```python
from build123d import *

# Parameters (mm, degrees)
F0_R     = 1.524
F1_DEPTH = 3.175
F2_R     = 5.08


# Not quite as in the source:
# - a feature names something its author has since deleted; it is built from what else it names


with BuildPart() as f1:
    # F0 (on Top) → F1 (new body)
    with BuildSketch(Plane.XY):
        Polygon((-6.35, -25.4), (6.35, -25.4), (6.35, 25.4), (6.35, 76.2), (-6.35, 76.2), (-6.35, 25.4), align=None)
        with Locations((0, -19.05)):
            Circle(F0_R, mode=Mode.SUBTRACT)
        with Locations((0, 19.05)):
            Circle(F0_R, mode=Mode.SUBTRACT)
    extrude(amount=F1_DEPTH)

    # F2
    f2_edges = [f1.edges().sort_by_distance(p)[0] for p in [
        (-6.35, 76.2, 1.5875),
        (6.35, 76.2, 1.5875),
        (-6.35, -25.4, 1.5875),
        (6.35, -25.4, 1.5875),
    ]]
    fillet(f2_edges, radius=F2_R)


solid = f1.part
```
Input: part model. Units: mm. Frame: model coordinates. Give positions to 0.01 mm unless a question says otherwise; leave off trailing zeros. Order: outer loops, then holes, each group sorted by start corner. A loop starts at its lowest first (then second) coordinate and runs counter-clockwise, first axis right, second up. Notation, with made-up numbers: (60, 46) - (80, 46) arc R25 ccw to (80, 61) - close; hole circle Ø6 at (76, 22.25). An arc over 180 degrees is marked (long way). Use a Markdown table: item, result.
(1) Section query A-A (y = -19.05). Output: boundary loops of the cut face in (x, z) (3 decimals), then the cut area to 3 significant figures.
Computed values:
| item | result |
|---|---|
| outline | (-6.35, 0) - (-1.524, 0) - (-1.524, 3.175) - (-6.35, 3.175) - close; (1.524, 0) - (6.35, 0) - (6.35, 3.175) - (1.524, 3.175) - close |
| area | 30.6 mm2 |
(2) Section query C-C (z = 1). Output: boundary loops of the cut face in (x, y), then the cut area to 3 significant figures.
Computed values:
| item | result |
|---|---|
| outline | (-6.35, -20.32) arc R5.08 ccw to (-1.27, -25.4) - (1.27, -25.4) arc R5.08 ccw to (6.35, -20.32) - (6.35, 71.12) arc R5.08 ccw to (1.27, 76.2) - (-1.27, 76.2) arc R5.08 ccw to (-6.35, 71.12) - close; hole circle Ø3.05 at (0, -19.05); hole circle Ø3.05 at (0, 19.05) |
| area | 1,250 mm2 |
(3) Section query D-D (x = 4). Output: boundary loops of the cut face in (y, z) (3 decimals), then the cut area to 3 significant figures.
Computed values:
| item | result |
|---|---|
| outline | (-24.604, 0) - (75.404, 0) - (75.404, 3.175) - (-24.604, 3.175) - close |
| area | 318 mm2 |
(4) Line query: line 1 (Y direction, x = 0, z = 1.7); line 2 (Y direction, x = -0.75, z = 2.65); line 3 (Y direction, x = 5, z = 2.8). Output: solid intervals per line, ascending. Write a range as from..to.
Computed values:
| item | result |
|---|---|
| line 1 | y = -25.4..-20.57, -17.53..17.53, 20.57..76.2 |
| line 2 | y = -25.4..-20.38, -17.72..17.72, 20.38..76.2 |
| line 3 | y = -23.77..74.57 |
(5) Section query B-B (x = 0). Output: boundary loops of the cut face in (y, z) (3 decimals).
Computed values:
| item | result |
|---|---|
| outline | (-25.4, 0) - (-20.574, 0) - (-20.574, 3.175) - (-25.4, 3.175) - close; (-17.526, 0) - (17.526, 0) - (17.526, 3.175) - (-17.526, 3.175) - close; (20.574, 0) - (76.2, 0) - (76.2, 3.175) - (20.574, 3.175) - close |
(6) Draft query along X for faces 1 (the cylindrical face through (-0.33, -20.538, 1.565)), 2 (the flat face through (0, 76.2, 2)), 3 (the cylindrical face through (-4.822, -23.951, 1.61)). Return one class per face: released by +X, released by -X, zero draft, split by the parting line, or undercut.
Computed values:
| item | result |
|---|---|
| face 1 | undercut |
| face 2 | zero draft |
| face 3 | released by -X |
